```python
from build123d import *

# Parameters (mm, degrees)
BOSS_EXTRUDE2_DEPTH = 11.75
SKETCH5_W           = 15.5
SKETCH5_H           = 5.5
CUT_EXTRUDE2_DEPTH  = 56.302011717
FILLET1_R           = 1
SKETCH7_R           = 10.25
CUT_EXTRUDE3_DEPTH  = 7.5


with BuildPart() as part:
    # Sketch1 → Boss-Extrude2 (new, symmetric)
    with BuildSketch(Plane.XY):
        with BuildLine():
            Line((-25, 6.5), (-25, -5))
            ThreePointArc((-25, -5), (-24.707106781, -5.707106781), (-24, -6))
            Line((-24, -6), (-18, -6))
            ThreePointArc((-18, -6), (-17.292893219, -6.292893219), (-17, -7))
            Line((-17, -7), (-17, -13))
            ThreePointArc((-17, -13), (-16.707106781, -13.707106781), (-16, -14))
            Line((-16, -14), (-4, -14))
            Line((-4, -14), (8, -14))
            ThreePointArc((8, -14), (8.707106781, -13.707106781), (9, -13))
            Line((9, -13), (9, -7))
            ThreePointArc((9, -7), (9.292893219, -6.292893219), (10, -6))
            Line((10, -6), (16, -6))
            ThreePointArc((16, -6), (16.707106781, -6.292893219), (17, -7))
            Line((17, -7), (17, -11))
            Line((17, -11), (17, -13))
            ThreePointArc((17, -13), (17.292893219, -13.707106781), (18, -14))
            Line((18, -14), (24, -14))
            ThreePointArc((24, -14), (24.707106781, -13.707106781), (25, -13))
            Line((25, -13), (25, -12))
            ThreePointArc((25, -12), (24.707106781, -11.292893219), (24, -11))
            Line((24, -11), (23, -11))
            ThreePointArc((23, -11), (22.292893219, -10.707106781), (22, -10))
            Line((22, -10), (22, -7))
            ThreePointArc((22, -7), (22.292893219, -6.292893219), (23, -6))
            Line((23, -6), (24, -6))
            ThreePointArc((24, -6), (24.707106781, -5.707106781), (25, -5))
            Line((25, -5), (25, 8.5))
            Line((25, 8.5), (25, 16))
            Line((25, 16), (25, 19.5))
            ThreePointArc((25, 19.5), (24.707106781, 20.207106781), (24, 20.5))
            Line((24, 20.5), (18, 20.5))
            ThreePointArc((18, 20.5), (17.292893219, 20.207106781), (17, 19.5))
            Line((17, 19.5), (17, 18.5))
            ThreePointArc((17, 18.5), (17.292893219, 17.792893219), (18, 17.5))
            Line((18, 17.5), (19, 17.5))
            ThreePointArc((19, 17.5), (19.707106781, 17.207106781), (20, 16.5))
            Line((20, 16.5), (20, 8.5))
            ThreePointArc((20, 8.5), (19.707106781, 7.792893219), (19, 7.5))
            Line((19, 7.5), (-24, 7.5))
            ThreePointArc((-24, 7.5), (-24.707106781, 7.207106781), (-25, 6.5))
        make_face()
    extrude(amount=BOSS_EXTRUDE2_DEPTH, both=True)

    # Sketch5 → Cut-Extrude2 (cut, through all)
    with BuildSketch(Plane.ZY.offset(25)):
        with Locations((0, 0.75)):
            Rectangle(SKETCH5_W, SKETCH5_H)
    extrude(amount=-CUT_EXTRUDE2_DEPTH, mode=Mode.SUBTRACT)

    # Fillet1
    fillet1_edges = [part.edges().sort_by_distance(p)[0] for p in [
        (-25, 3.5, 0),
        (25, -2, 0),
        (25, 3.5, 0),
        (-25, -2, 0),
    ]]
    fillet(fillet1_edges, radius=FILLET1_R)

    # Sketch7 → Cut-Extrude3 (cut, symmetric)
    with BuildSketch(Plane.XZ.offset(14)):
        with Locations(Location((-4, 0, 0), (0, 0, 270))):
            Circle(SKETCH7_R)
    extrude(amount=CUT_EXTRUDE3_DEPTH, both=True, mode=Mode.SUBTRACT)


solid = part.part
```
Check sheet for the modelled part. Datum: model origin and axes. Units: mm. A direction names the side the tool comes from. Round coordinates to 2 decimals unless told otherwise and drop trailing zeros. Order: outer loops, then holes, each group sorted by start corner. A loop starts at its lowest first (then second) coordinate and runs counter-clockwise, first axis right, second up. Notation, with made-up numbers: (-38.75, 6) - (-19.75, 6) arc R33 cw to (-19.75, 44) - close; hole circle Ø5 at (-2, -22.75). An arc over 180 degrees is marked (long way). Answer as CSV lines item,"result". Start each with the question number.
1) Section check C-C (y = 1). Record the cut outline in (x, z).
2) Draft check along X on faces 6 (the face through (0, 1, 7.75)), 7 (the face through (19.715, 7.801, 0.165)), 8 (the face through (17, -10, 0)). Enter one of: +X half, -X half, draft (parallel to the pull), parting line (faces both ways), or undercut.
3) Section check A-A (y = -8.5). Record the cut outline in (x, z).
4) Section check B-B (x = -4). Record the cut outline in (y, z).
5) Scan lines: probe 1 along X at (y, z) = (-8.5, 0); probe 2 along Y at (x, z) = (-8, 1); probe 3 along Y at (x, z) = (-20, 3.25). Record each from-to range of solid material in increasing order.
6) Section check D-D (x = 13.5). Record the cut outline in (y, z), then the cut area to 3 significant figures.
7) Tool access check on faces 1 (the face through (24.715, -11.301, 0.165)), 2 (the face through (-21, -6, 0)), 3 (the face through (18.5, 17.5, 0.2)), 4 (the face through (24.699, -2.285, -0.109)), 5 (the face through (0, 3.5, 0)). Record the directions out of +Z, -Z, +X, -X, +Y, -Y that give a thin tool (end or side, any length) a straight path to the whole face; none if there is none.
8) Depth check by flat-ended pin: pin 1 (3 mm diameter, centred on x = -20.5, z = 4, fed in from -Y); pin 2 (5 mm diameter, centred on x = -15, z = -3.5, fed in from +Y); pin 3 (0.8 mm diameter, centred on y = 19, z = 2, fed in from -X). Enter the tip coordinate at first touch or a pass-through.
Determined:
1,outline,"(-25, -11.75) - (25, -11.75) - (25, -7.75) - (-25, -7.75) - close; (-25, 7.75) - (25, 7.75) - (25, 11.75) - (-25, 11.75) - close"
2,face 6,"draft"
2,face 7,"-X half"
2,face 8,"undercut"
3,outline,"(-17, -11.75) - (9, -11.75) - (9, 11.75) - (-17, 11.75) - close; (17, -11.75) - (22, -11.75) - (22, 11.75) - (17, 11.75) - close; hole circle Ø20.5 at (-4, 0)"
4,outline,"(-14, -11.75) - (7.5, -11.75) - (7.5, 11.75) - (-14, 11.75) - (-14, 10.25) - (-6.5, 10.25) - (-6.5, -10.25) - (-14, -10.25) - close; hole (-2, -7.75) - (3.5, -7.75) - (3.5, 7.75) - (-2, 7.75) - close"
5,probe 1,"-17 to -14.25, 6.25 to 9, 17 to 22"
5,probe 2,"-6.5 to -2, 3.5 to 7.5"
5,probe 3,"-6 to -2, 3.5 to 7.5"
6,outline,"(-6, -11.75) - (7.5, -11.75) - (7.5, 11.75) - (-6, 11.75) - close; hole (-2, -7.75) - (3.5, -7.75) - (3.5, 7.75) - (-2, 7.75) - close"
6,area,"232 mm^2"
7,face 1,"+Z, -Z, +X"
7,face 2,"+Z, -Z, -X, -Y"
7,face 3,"+Z, -Z, -X"
7,face 4,"+X"
7,face 5,"+X, -X"
8,pin 1,"y = -6"
8,pin 2,"y = 7.5"
8,pin 3,"x = 17"
